Check sheet for the modelled part. Datum: model origin and axes. Units: mm. Face numbers are marked on the shaded views. A direction names the side the tool comes from. Give positions to 0.01 mm unless a question says otherwise; leave off trailing zeros. Loops run counter-clockwise (first coordinate to the right, second up) from the corner with the lowest first, then second, coordinate; pieces in that order, holes last. Notation, with made-up numbers: (13, 62) - (72, 62) arc R26 ccw to (72, 84) - close; hole circle Ø11 at (55, 53). An arc over 180 degrees is marked (long way). Use one line per item in the form item = value.
from build123d import *

# Parameters (mm, degrees)
F2_W      = 60
F2_H      = 8
F2_R      = 3
F5_DEPTH  = 5
F1_R      = 3
F1_R_2    = 1.7
F6_DEPTH  = 4
F0_R      = 1.7
F7_DEPTH  = 12.5
F3_R      = 2.05
F8_DEPTH  = 2
F9_DEPTH  = 2
F11_DEPTH = 2.4
F12_R     = 3.99999
F4_R      = 1.2
F13_DEPTH = 5.001


# Not quite as in the source:
# - a fillet or chamfer is up to 0.001 mm smaller than in the source, because OpenCascade refuses the exact size


with BuildPart() as f5:
    # F2 (on face) → F5 (new body)
    with BuildSketch(Plane.XY):
        with Locations((0, 38)):
            Rectangle(F2_W, F2_H)
        with Locations((-26, 38)):
            Circle(F2_R, mode=Mode.SUBTRACT)
        Polygon((1.1402667816, 36.025), (0, 36.025), (-1.1402667816, 36.025), (-2.2805335633, 38), (-1.1402667816, 39.975), (0, 39.975), (1.1402667816, 39.975), (2.2805335633, 38), align=None, mode=Mode.SUBTRACT)
        with Locations((26, 38)):
            Circle(F2_R, mode=Mode.SUBTRACT)
        Polygon((-1.1402667816, 36.025), (0, 36.025), (1.1402667816, 36.025), (2.2805335633, 38), (1.1402667816, 39.975), (0, 39.975), (-1.1402667816, 39.975), (-2.2805335633, 38), align=None)
        with Locations((-26, 38)):
            Circle(F2_R)
        with Locations((26, 38)):
            Circle(F2_R)
    extrude(amount=F5_DEPTH)

    # F1 (on Top) → F6 (join)
    with BuildSketch(Plane.XY):
        with Locations((-26, 38)):
            Circle(F1_R)
        with Locations((-26, 38)):
            Circle(F1_R_2, mode=Mode.SUBTRACT)
        with Locations((26, 38)):
            Circle(F1_R)
        with Locations((26, 38)):
            Circle(F1_R_2, mode=Mode.SUBTRACT)
    extrude(amount=-F6_DEPTH)

    # F0 (on Top) → F7 (cut, symmetric)
    with BuildSketch(Plane.XY):
        with Locations((-26, 38)):
            Circle(F0_R)
        with Locations((26, 38)):
            Circle(F0_R)
        with Locations((-26, -38)):
            Circle(F0_R)
        with Locations((26, -38)):
            Circle(F0_R)
    extrude(amount=F7_DEPTH, both=True, mode=Mode.SUBTRACT)

    # F3 (on face) → F8 (cut)
    with BuildSketch(Plane.XY):
        with Locations((-7.225, 38)):
            Circle(F3_R)
        with Locations((7.225, 38)):
            Circle(F3_R)
    extrude(amount=F8_DEPTH, mode=Mode.SUBTRACT)

    # F2 (on face) → F9 (cut)
    with BuildSketch(Plane.XY):
        Polygon((-1.1402667816, 36.025), (0, 36.025), (1.1402667816, 36.025), (2.2805335633, 38), (1.1402667816, 39.975), (0, 39.975), (-1.1402667816, 39.975), (-2.2805335633, 38), align=None)
    extrude(amount=F9_DEPTH, mode=Mode.SUBTRACT)

    # F10 (on face) → F11 (cut)
    with BuildSketch(Plane.XY.offset(5)):
        Polygon((-27.5732794835, 35.275), (-26, 35.275), (-24.4267205165, 35.275), (-22.8534410329, 38), (-24.4267205165, 40.725), (-26, 40.725), (-27.5732794835, 40.725), (-29.1465589671, 38), align=None)
        Polygon((22.8534410329, 38), (24.4267205165, 35.275), (26, 35.275), (27.5732794835, 35.275), (29.1465589671, 38), (27.5732794835, 40.725), (26, 40.725), (24.4267205165, 40.725), align=None)
    extrude(amount=-F11_DEPTH, mode=Mode.SUBTRACT)

    # F12 (radius 4 in the source; OpenCascade refuses exactly that, so slightly less here)
    f12_edges = [f5.edges().sort_by_distance(p)[0] for p in [
        (-30, 42, 2.5),
        (-30, 34, 2.5),
        (30, 42, 2.5),
        (30, 34, 2.5),
    ]]
    fillet(f12_edges, radius=F12_R)

    # F4 (on face) → F13 (cut, through all)
    with BuildSketch(Plane.XY):
        with Locations((-7.225, 38)):
            Circle(F4_R)
        with Locations((0, 38)):
            Circle(F4_R)
        with Locations((7.225, 38)):
            Circle(F4_R)
    extrude(amount=F13_DEPTH, mode=Mode.SUBTRACT)


solid = f5.part
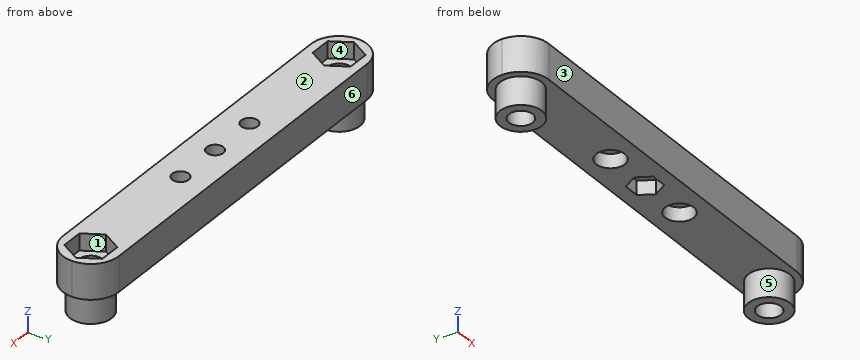
Item 1: Section check D-D on y = 41.5. Record the boundary of the cut face in (x, z).
Answer block:
outline = (-27.94, 0) - (27.94, 0) - (27.94, 5) - (-27.94, 5) - close
Item 2: Mould release check, pull along Y, two halves, no side actions. Record for the marked faces 1, 2 and 3: released by +Y, released by -Y, zero draft, split by the parting line, or undercut.
Answer block:
face_1 = undercut
face_2 = zero draft
face_3 = released by -Y
Item 3: Gauge pin test, flat ends, axial feed: P1, Ø1.5, axis at x = 19.5, y = 39.5, coming from the -Z side; P2, Ø1.5, axis at y = 35, z = 0.5, coming from the -X side; P3, Ø1.9, axis at x = -7.225, y = 38, coming from the +Z side; P4, Ø1.2, axis at x = 8, y = 39, coming from the -Z side. Record the tip position at first contact, or that the pin passes through.
Answer block:
P1 = 0
P2 = -29.31
P3 = through
P4 = 2
Item 4: Access from +Z, -Z, +X, -X, +Y, -Y to the whole of each face (thin tool, end or side, straight path). Record for the marked faces 4, 5 and 6.
Answer block:
face_4 = +Z
face_5 = -Z
face_6 = +Z, -Z, +X, -X, +Y
Item 5: Section check B-B on z = 4.25. Give the number of separate pieces and of enclosed holes in the cut face, then the cut area to 3 significant figures.
Answer block:
separate_pieces = 1
enclosed_holes = 5
area = 401 mm2
Item 6: Section check A-A on z = -1.5. Record the boundary of the cut face in (x, y).
Answer block:
outline = circle Ø6 at (-26, 38); circle Ø6 at (26, 38); hole circle Ø3.4 at (-26, 38); hole circle Ø3.4 at (26, 38)
Item 7: Thickness scan on L1, parallel to X at y = 38, z = 3.1 (3 decimals); L2, parallel to X at y = 36.75, z = 1.5; L3, parallel to Y at x = 0, z = 3.8. Record the ranges inside material, lowest first.
Answer block:
L1 = -30 to -29.147, -22.853 to -8.425, -6.025 to -1.2, 1.2 to 6.025, 8.425 to 22.853, 29.147 to 30
L2 = -29.8 to -27.15, -24.85 to -8.85, -5.6 to -1.56, 1.56 to 5.6, 8.85 to 24.85, 27.15 to 29.8
L3 = 34 to 36.8, 39.2 to 42
Item 8: Section check C-C on x = 0. Record the boundary of the cut face in (y, z) (3 decimals).
Answer block:
outline = (34, 0) - (36.025, 0) - (36.025, 2) - (36.8, 2) - (36.8, 5) - (34, 5) - close; (39.2, 2) - (39.975, 2) - (39.975, 0) - (42, 0) - (42, 5) - (39.2, 5) - close
